Can you work these out from the model? Positions are in its coordinate system, mm. A direction names the side the tool comes from. Give positions to 0.01 mm unless a question says otherwise; leave off trailing zeros. Write each loop counter-clockwise with the first axis right and the second up, starting at its lowest first coordinate (ties: lowest second). Pieces come first, ordered by that corner, then holes.
from build123d import *

# Parameters (mm, degrees)
SKETCH1_W           = 1498.6
SKETCH1_H           = 50.8
BOSS_EXTRUDE1_DEPTH = 25.4
CUT_EXTRUDE1_DEPTH  = 1498.6
CUT_EXTRUDE2_DEPTH  = 1499.869043646
CUT_EXTRUDE3_DEPTH  = 1498.6
CUT_EXTRUDE4_DEPTH  = 1498.6
CUT_EXTRUDE5_DEPTH  = 1499.869043646
CUT_EXTRUDE6_DEPTH  = 1499.869043646
CUT_EXTRUDE7_DEPTH  = 1498.6
CUT_EXTRUDE8_DEPTH  = 1498.6
SKETCH10_W          = 20.32
SKETCH10_H          = 45.72
CUT_EXTRUDE9_DEPTH  = 1499.869043646
DRAFT1_ANGLE        = 45
DRAFT2_ANGLE        = 45.000000005
DRAFT3_ANGLE        = 45
DRAFT4_ANGLE        = 45
DRAFT5_ANGLE        = 45
DRAFT6_ANGLE        = 44.999999995
SKETCH11_W          = 61.962293059
SKETCH11_H          = 88.678950317
CUT_EXTRUDE10_DEPTH = 1371.6
SKETCH13_R          = 6.35
CUT_EXTRUDE11_DEPTH = 25.4


with BuildPart() as part:
    # Sketch1 → Boss-Extrude1 (new body)
    with BuildSketch(Plane(origin=(12.7, 0, 0), x_dir=(0, 0, -1), z_dir=(1, 0, 0))):
        Rectangle(SKETCH1_W, SKETCH1_H)
    extrude(amount=-BOSS_EXTRUDE1_DEPTH)

    # Sketch2 → Cut-Extrude1 (cut)
    with BuildSketch(Plane.XY.offset(749.3)):
        Polygon((0.0762, 25.4), (-0.0762, 25.4), (0.0762, 25.2476), align=None)
    extrude(amount=-CUT_EXTRUDE1_DEPTH, mode=Mode.SUBTRACT)

    # Sketch3 → Cut-Extrude2 (cut, through all)
    with BuildSketch(Plane.XY.offset(749.3)):
        Polygon((12.7, 12.6238), (12.7, 12.7762), (12.5476, 12.7762), align=None)
    extrude(amount=-CUT_EXTRUDE2_DEPTH, mode=Mode.SUBTRACT)

    # Sketch4 → Cut-Extrude3 (cut)
    with BuildSketch(Plane.XY.offset(749.3)):
        Polygon((12.7, -0.0762), (12.7, 0.0762), (12.5476, -0.0762), align=None)
    extrude(amount=-CUT_EXTRUDE3_DEPTH, mode=Mode.SUBTRACT)

    # Sketch5 → Cut-Extrude4 (cut)
    with BuildSketch(Plane.XY.offset(749.3)):
        Polygon((12.7, -12.7762), (12.7, -12.6238), (12.5476, -12.6238), align=None)
    extrude(amount=-CUT_EXTRUDE4_DEPTH, mode=Mode.SUBTRACT)

    # Sketch6 → Cut-Extrude5 (cut, through all)
    with BuildSketch(Plane.XY.offset(749.3)):
        Polygon((0.0762, -25.4), (-0.0762, -25.2476), (-0.0762, -25.4), align=None)
    extrude(amount=-CUT_EXTRUDE5_DEPTH, mode=Mode.SUBTRACT)

    # Sketch7 → Cut-Extrude6 (cut, through all)
    with BuildSketch(Plane.XY.offset(749.3)):
        Polygon((-12.7, -12.6238), (-12.7, -12.7762), (-12.5476, -12.7762), align=None)
    extrude(amount=-CUT_EXTRUDE6_DEPTH, mode=Mode.SUBTRACT)

    # Sketch8 → Cut-Extrude7 (cut)
    with BuildSketch(Plane.XY.offset(749.3)):
        Polygon((-12.7, 0.0762), (-12.7, -0.0762), (-12.5476, 0.0762), align=None)
    extrude(amount=-CUT_EXTRUDE7_DEPTH, mode=Mode.SUBTRACT)

    # Sketch9 → Cut-Extrude8 (cut)
    with BuildSketch(Plane.XY.offset(749.3)):
        Polygon((-12.7, 12.7762), (-12.7, 12.6238), (-12.5476, 12.6238), align=None)
    extrude(amount=-CUT_EXTRUDE8_DEPTH, mode=Mode.SUBTRACT)

    # Sketch10 → Cut-Extrude9 (cut, through all)
    with BuildSketch(Plane.XY.offset(749.3)):
        Rectangle(SKETCH10_W, SKETCH10_H)
    extrude(amount=-CUT_EXTRUDE9_DEPTH, mode=Mode.SUBTRACT)

    # Draft1
    draft1_faces = [part.faces().sort_by_distance(p)[0] for p in [
        (0.0762, 25.3238, 0),
    ]]
    draft(draft1_faces, Plane(origin=(-12.7, 25.4, -749.3), x_dir=(0, 0, 1), z_dir=(0, 1, 0)), DRAFT1_ANGLE)

    # Draft2
    draft2_faces = [part.faces().sort_by_distance(p)[0] for p in [
        (12.6238, 12.7762, 0),
    ]]
    draft(draft2_faces, Plane(origin=(12.7, 0, 0), x_dir=(0, 0, 1), z_dir=(1, 0, 0)), DRAFT2_ANGLE)

    # Draft3
    draft3_faces = [part.faces().sort_by_distance(p)[0] for p in [
        (-0.0762, -25.3238, 0),
    ]]
    draft(draft3_faces, Plane(origin=(-12.7, -25.4, 749.3), x_dir=(0, 0, -1), z_dir=(0, -1, 0)), DRAFT3_ANGLE)

    # Draft4
    draft4_faces = [part.faces().sort_by_distance(p)[0] for p in [
        (-12.6238, -12.7762, 0),
    ]]
    draft(draft4_faces, Plane(origin=(-12.7, 0, 0), x_dir=(0, 0, -1), z_dir=(-1, 0, 0)), DRAFT4_ANGLE)

    # Draft5
    draft5_faces = [part.faces().sort_by_distance(p)[0] for p in [
        (12.6238, -12.6238, 0),
        (12.6238, 0, 0),
    ]]
    draft(draft5_faces, Plane(origin=(12.7, 0, 0), x_dir=(0, 0, 1), z_dir=(1, 0, 0)), DRAFT5_ANGLE)

    # Draft6
    draft6_faces = [part.faces().sort_by_distance(p)[0] for p in [
        (-12.6238, 0, 0),
        (-12.6238, 12.6238, 0),
    ]]
    draft(draft6_faces, Plane(origin=(-12.7, 0, 0), x_dir=(0, 0, -1), z_dir=(-1, 0, 0)), DRAFT6_ANGLE)

    # Sketch11 → Cut-Extrude10 (cut)
    with BuildSketch(Plane(origin=(0, 0, -749.3), x_dir=(-1, 0, 0), z_dir=(0, 0, -1))):
        with Locations((-2.92473676, 0.325700182)):
            Rectangle(SKETCH11_W, SKETCH11_H)
    extrude(amount=-CUT_EXTRUDE10_DEPTH, mode=Mode.SUBTRACT)

    # Sketch13 → Cut-Extrude11 (cut)
    with BuildSketch(Plane(origin=(12.7, 0, 0), x_dir=(0, 0, -1), z_dir=(1, 0, 0))):
        with Locations((-723.9, 0.0762)):
            Circle(SKETCH13_R)
    extrude(amount=-CUT_EXTRUDE11_DEPTH, mode=Mode.SUBTRACT)


solid = part.part
(1) Will these pins go through, and if not, where does the flat tip stop? P1, Ø16.5, axis at y = 0.08, z = 723.9, coming from the +X side; P2, Ø10, axis at x = -4, y = -2.5, coming from the -Z side (3 decimals).
Returned:
P1: stops at x = 12.7
P2: passes through
(2) If I drill on L1, parallel to X at y = 5, z = 663.5; L2, parallel to Y at x = -3, z = 671; L3, parallel to Y at x = -11.6, z = 723.9, over which ranges is the centre line in solid material (lowest first)?
Returned:
L1: x = -12.7 to -10.16, 10.16 to 12.7
L2: y = -25.4 to -22.86, 22.86 to 25.4
L3: y = -25.4 to -6.27, 6.43 to 25.4
(3) Imagine slicing it at C-C, the plane y = 19. Write out the boundary of the cut face in (x, z), plus the area to 3 significant figures.
Returned:
outline: (-12.7, 622.3) - (-10.16, 622.3) - (-10.16, 749.3) - (-12.7, 749.3) - close; (10.16, 622.3) - (12.7, 622.3) - (12.7, 749.3) - (10.16, 749.3) - close
area: 645 mm2
(4) If we mould it in two halves opening along Y, with no side actions, what happens to faces 3 (the face through (-11.412, 0.355, 730.244)), 4 (the face through (6, -25.4, 687)), 5 (the face through (12.7, 19, 687))? For each: +Y half, -Y half, draft (parallel to the pull), parting line (faces both ways), or undercut.
Returned:
face 3: undercut
face 4: -Y half
face 5: draft
(5) Imagine slicing it at A-A, the plane x = -4.25. Write out the boundary of the cut face in (y, z).
Returned:
outline: (-25.4, 622.3) - (-22.86, 622.3) - (-22.86, 749.3) - (-25.4, 749.3) - close; (22.86, 622.3) - (25.4, 622.3) - (25.4, 749.3) - (22.86, 749.3) - close
(6) For faces 1 (the face through (11.448, 0.355, 730.244)), 2 (the face through (0, -22.86, 687)), which set-ups out of +Z, -Z, +X, -X, +Y, -Y let a thin tool reach every point of the face, with its end or its side?
Returned:
face 1: +X, -X
face 2: +Z, -Z
